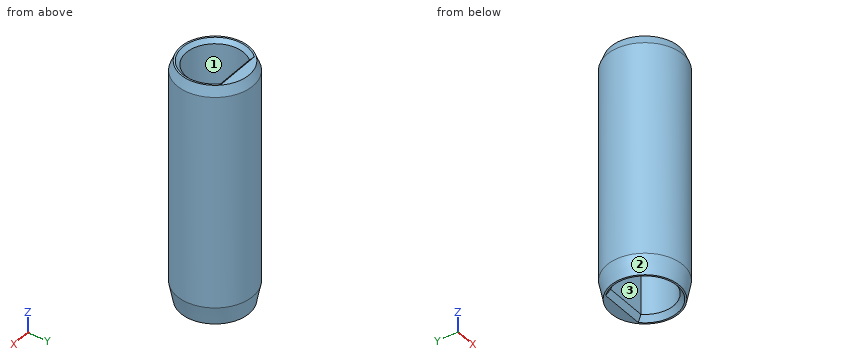
```python
from build123d import *

# Parameters (mm, degrees)
F0_R     = 2
F1_DEPTH = 12.7
F2_SIZE2 = 0.2
F2_SIZE  = 1
F3_SIZE2 = 0.5
F3_SIZE  = 0.2
F4_SIZE  = 0.2
F5_SIZE2 = 0.3
F5_SIZE  = 0.2


with BuildPart() as f1:
    # F0 (on Top) → F1 (new body)
    with BuildSketch(Plane.XY):
        Circle(F0_R)
        with BuildLine():
            ThreePointArc((1.1213524201, 1.015), (1.411329477, 0.5438799108), (1.5125, 0))
            ThreePointArc((1.5125, 0), (-0.5438799108, -1.411329477), (-1.1213524201, 1.015))
            ThreePointArc((-1.1213524201, 1.015), (0, 1.5125), (1.1213524201, 1.015))
        make_face(mode=Mode.SUBTRACT)
        with BuildLine():
            Line((0, 1.015), (1.1213524201, 1.015))
            ThreePointArc((1.1213524201, 1.015), (0, 1.5125), (-1.1213524201, 1.015))
            Line((-1.1213524201, 1.015), (0, 1.015))
        make_face()
    extrude(amount=F1_DEPTH)

    # F2
    f2_edges = [f1.edges().sort_by_distance(p)[0] for p in [
        (-2, 0, 0),
    ]]
    f2_side = f1.faces().sort_by_distance((-2, 0, 6.35))[0]
    chamfer(f2_edges, length=F2_SIZE, length2=F2_SIZE2, reference=f2_side)

    # F3
    f3_edges = [f1.edges().sort_by_distance(p)[0] for p in [
        (-2, 0, 12.7),
    ]]
    f3_side = f1.faces().sort_by_distance((-1.943431, 0, 12.7))[0]
    chamfer(f3_edges, length=F3_SIZE, length2=F3_SIZE2, reference=f3_side)

    # F4
    f4_edges = [f1.edges().sort_by_distance(p)[0] for p in [
        (0, 1.015, 12.7),
        (0, -1.5125, 12.7),
    ]]
    chamfer(f4_edges, length=F4_SIZE)

    # F5
    f5_edges = [f1.edges().sort_by_distance(p)[0] for p in [
        (0, -1.5125, 0),
        (0, 1.015, 0),
    ]]
    f5_side = f1.faces().sort_by_distance((-1.749088, 0, 0))[0]
    chamfer(f5_edges, length=F5_SIZE, length2=F5_SIZE2, reference=f5_side)


solid = f1.part
```
Source: CAD feature listing. Evaluate the final solid. Frame: model axes, mm. Face numbers are marked on the shaded views. Round coordinates to 2 decimals unless told otherwise and drop trailing zeros. Loops run counter-clockwise (first coordinate to the right, second up) from the corner with the lowest first, then second, coordinate; pieces in that order, holes last.
(1) Material intervals for probe 1 along Y at (x, z) = (0, 6.25) (1 decimal); probe 2 along X at (y, z) = (0.1, 2); probe 3 along Y at (x, z) = (-1.2, 12), sorted ascending.
From the geometry:
probe 1: y = -2 to -1.5, 1 to 2
probe 2: x = -2 to -1.51, 1.51 to 2
probe 3: y = -1.6 to -0.92, 0.92 to 1.6
(2) Section query C-C (z = 7.5). Output: boundary loops of the cut face in (x, y) (1 decimal).
From the geometry:
outline: circle Ø4 at (0, 0); hole (-1.1, 1) arc R1.5 ccw (long way) to (1.1, 1) - close
(3) Section query B-B (y = 0). Output: boundary loops of the cut face in (x, z), and give its area (3 significant figures).
From the geometry:
outline: (-2, 1) - (-1.8, 0) - (-1.71, 0) - (-1.51, 0.3) - (-1.51, 12.5) - (-1.71, 12.7) - (-1.8, 12.7) - (-2, 12.2) - close; (1.51, 0.3) - (1.71, 0) - (1.8, 0) - (2, 1) - (2, 12.2) - (1.8, 12.7) - (1.71, 12.7) - (1.51, 12.5) - close
area: 12.0 mm2
(4) Pull-direction query (Y, two-part tool) for the marked faces 1, 2 and 3; classes: +Y half, -Y half, draft (parallel to the pull), parting line (faces both ways), or undercut.
From the geometry:
face 1: undercut
face 2: parting line
face 3: undercut
(5) Contact query for flat-ended pins moving along their axis: pin 1 Ø1.5 at (y, z) = (1, 7) entering from +X; pin 2 Ø1.5 at (x, z) = (1, 7) entering from -Y. Output: stop coordinate, or through.
From the geometry:
pin 1: stops at x = 1.98
pin 2: stops at y = -1.98
